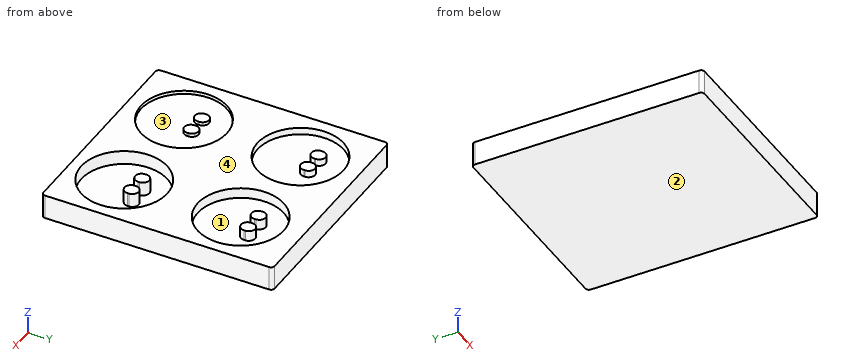
from build123d import *

# Parameters (mm, degrees)
BOSS_EXTRUDE1_DEPTH = 7
CAVITY1_START       = -3
CAVITY1_OUTLINE_R   = 12.36
CAVITY1_DEPTH       = 3
CAVITY1_START_2     = -2
CAVITY1_2_OUTLINE_R = 12.36
CAVITY1_2_DEPTH     = 2
CAVITY1_START_3     = -4
CAVITY1_3_OUTLINE_R = 12.36
CAVITY1_3_DEPTH     = 1
CAVITY1_START_4     = -1
CAVITY1_4_OUTLINE_R = 12.36
CAVITY1_4_DEPTH     = 1


# Read off the part's stored shape, not the designer's step: Cavity1
with BuildPart() as part:
    # Sketch1 → Boss-Extrude1 (new body)
    with BuildSketch(Plane.XY):
        with BuildLine():
            Line((38.123582206, -19.216804324), (-21.063563238, -19.216804324))
            ThreePointArc((-21.063563238, -19.216804324), (-21.770670019, -18.923911105), (-22.063563238, -18.216804324))
            Line((-22.063563238, -18.216804324), (-22.063563238, 46.15189529))
            ThreePointArc((-22.063563238, 46.15189529), (-21.770670019, 46.859002071), (-21.063563238, 47.15189529))
            Line((-21.063563238, 47.15189529), (38.123582206, 47.15189529))
            ThreePointArc((38.123582206, 47.15189529), (38.830688987, 46.859002071), (39.123582206, 46.15189529))
            Line((39.123582206, 46.15189529), (39.123582206, -18.216804324))
            ThreePointArc((39.123582206, -18.216804324), (38.830688987, -18.923911105), (38.123582206, -19.216804324))
        make_face()
    extrude(amount=-BOSS_EXTRUDE1_DEPTH)

    # Cavity1 outline → Cavity1 (cut)
    # profile 1 of 2: a face of its own
    with BuildSketch(Plane.XY.offset(CAVITY1_START)):
        with Locations((23.634896534, -3.890788044)):
            Circle(CAVITY1_OUTLINE_R)
        with BuildLine():
            ThreePointArc((18.999896534, -0.040788044), (20.849896534, 1.809211956), (22.699896534, -0.040788044))
            Line((22.699896534, -0.040788044), (22.699896534, -0.430788044))
            ThreePointArc((22.699896534, -0.430788044), (20.849896534, -2.280788044), (18.999896534, -0.430788044))
            Line((18.999896534, -0.430788044), (18.999896534, -0.040788044))
        make_face(mode=Mode.SUBTRACT)
        with BuildLine():
            ThreePointArc((24.569896534, -0.040788044), (26.419896534, 1.809211956), (28.269896534, -0.040788044))
            Line((28.269896534, -0.040788044), (28.269896534, -0.430788044))
            ThreePointArc((28.269896534, -0.430788044), (26.419896534, -2.280788044), (24.569896534, -0.430788044))
            Line((24.569896534, -0.430788044), (24.569896534, -0.040788044))
        make_face(mode=Mode.SUBTRACT)
    # profile 2 of 2: a face of its own
    with BuildSketch(Plane.XY.offset(CAVITY1_START)):
        with Locations((23.634896534, 29.54740971)):
            Circle(CAVITY1_OUTLINE_R)
        with BuildLine():
            Line((22.699896534, 33.39740971), (22.699896534, 33.00740971))
            ThreePointArc((22.699896534, 33.00740971), (20.849896534, 31.15740971), (18.999896534, 33.00740971))
            Line((18.999896534, 33.00740971), (18.999896534, 33.39740971))
            ThreePointArc((18.999896534, 33.39740971), (20.849896534, 35.24740971), (22.699896534, 33.39740971))
        make_face(mode=Mode.SUBTRACT)
        with BuildLine():
            Line((28.269896534, 33.39740971), (28.269896534, 33.00740971))
            ThreePointArc((28.269896534, 33.00740971), (26.419896534, 31.15740971), (24.569896534, 33.00740971))
            Line((24.569896534, 33.00740971), (24.569896534, 33.39740971))
            ThreePointArc((24.569896534, 33.39740971), (26.419896534, 35.24740971), (28.269896534, 33.39740971))
        make_face(mode=Mode.SUBTRACT)
    extrude(amount=CAVITY1_DEPTH, mode=Mode.SUBTRACT)

    # Cavity1 2 outline → Cavity1 2 (cut)
    with BuildSketch(Plane.XY.offset(CAVITY1_START_2)):
        with Locations((-6.365103466, 30.435007788)):
            Circle(CAVITY1_2_OUTLINE_R)
        with BuildLine():
            ThreePointArc((-11.000103466, 34.285007788), (-9.150103466, 36.135007788), (-7.300103466, 34.285007788))
            Line((-7.300103466, 34.285007788), (-7.300103466, 33.895007788))
            ThreePointArc((-7.300103466, 33.895007788), (-9.150103466, 32.045007788), (-11.000103466, 33.895007788))
            Line((-11.000103466, 33.895007788), (-11.000103466, 34.285007788))
        make_face(mode=Mode.SUBTRACT)
        with BuildLine():
            ThreePointArc((-5.430103466, 34.285007788), (-3.580103466, 36.135007788), (-1.730103466, 34.285007788))
            Line((-1.730103466, 34.285007788), (-1.730103466, 33.895007788))
            ThreePointArc((-1.730103466, 33.895007788), (-3.580103466, 32.045007788), (-5.430103466, 33.895007788))
            Line((-5.430103466, 33.895007788), (-5.430103466, 34.285007788))
        make_face(mode=Mode.SUBTRACT)
    extrude(amount=CAVITY1_2_DEPTH, mode=Mode.SUBTRACT)

    # Cavity1 3 outline → Cavity1 3 (cut)
    with BuildSketch(Plane.XY.offset(CAVITY1_START_3)):
        with Locations((23.634896534, -3.890788044)):
            Circle(CAVITY1_3_OUTLINE_R)
        with BuildLine():
            ThreePointArc((18.999896534, -0.040788044), (20.849896534, 1.809211956), (22.699896534, -0.040788044))
            Line((22.699896534, -0.040788044), (22.699896534, -0.430788044))
            ThreePointArc((22.699896534, -0.430788044), (20.849896534, -2.280788044), (18.999896534, -0.430788044))
            Line((18.999896534, -0.430788044), (18.999896534, -0.040788044))
        make_face(mode=Mode.SUBTRACT)
        with BuildLine():
            ThreePointArc((24.569896534, -0.040788044), (26.419896534, 1.809211956), (28.269896534, -0.040788044))
            Line((28.269896534, -0.040788044), (28.269896534, -0.430788044))
            ThreePointArc((28.269896534, -0.430788044), (26.419896534, -2.280788044), (24.569896534, -0.430788044))
            Line((24.569896534, -0.430788044), (24.569896534, -0.040788044))
        make_face(mode=Mode.SUBTRACT)
    extrude(amount=CAVITY1_3_DEPTH, mode=Mode.SUBTRACT)

    # Cavity1 4 outline → Cavity1 4 (cut)
    with BuildSketch(Plane.XY.offset(CAVITY1_START_4)):
        with Locations((-6.365103466, -3.03425393)):
            Circle(CAVITY1_4_OUTLINE_R)
        with BuildLine():
            Line((-7.300103466, 0.81574607), (-7.300103466, 0.42574607))
            ThreePointArc((-7.300103466, 0.42574607), (-9.150103466, -1.42425393), (-11.000103466, 0.42574607))
            Line((-11.000103466, 0.42574607), (-11.000103466, 0.81574607))
            ThreePointArc((-11.000103466, 0.81574607), (-9.150103466, 2.66574607), (-7.300103466, 0.81574607))
        make_face(mode=Mode.SUBTRACT)
        with BuildLine():
            Line((-1.730103466, 0.81574607), (-1.730103466, 0.42574607))
            ThreePointArc((-1.730103466, 0.42574607), (-3.580103466, -1.42425393), (-5.430103466, 0.42574607))
            Line((-5.430103466, 0.42574607), (-5.430103466, 0.81574607))
            ThreePointArc((-5.430103466, 0.81574607), (-3.580103466, 2.66574607), (-1.730103466, 0.81574607))
        make_face(mode=Mode.SUBTRACT)
    extrude(amount=CAVITY1_4_DEPTH, mode=Mode.SUBTRACT)


solid = part.part
Check sheet for the modelled part. Datum: model origin and axes. Units: mm. Face numbers are marked on the shaded views. A direction names the side the tool comes from. Round coordinates to 2 decimals unless told otherwise and drop trailing zeros. Write each loop counter-clockwise with the first axis right and the second up, starting at its lowest first coordinate (ties: lowest second). Pieces come first, ordered by that corner, then holes. Notation, with made-up numbers: (-0.75, -13) - (42.25, -13) arc R22 ccw to (42.25, 8) - close; hole circle Ø9 at (25, 40). An arc over 180 degrees is marked (long way). Return JSON: item names as keys, results as strings.
Q1. Access from +Z, -Z, +X, -X, +Y, -Y to the whole of each face (thin tool, end or side, straight path). Record for the marked faces 3 and 4.
Returned:
{"face 3": "+Z", "face 4": "+Z, +X, -X, +Y, -Y"}
Q2. Cross-section at D-D (x = -9). Record the boundary of the cut face in (y, z), then the cut area to 3 significant figures.
Returned:
{"outline": "(-19.22, -7) - (47.15, -7) - (47.15, 0) - (42.51, 0) - (42.51, -2) - (36.13, -2) - (36.13, 0) - (32.05, 0) - (32.05, -2) - (18.36, -2) - (18.36, 0) - (9.04, 0) - (9.04, -1) - (2.66, -1) - (2.66, 0) - (-1.42, 0) - (-1.42, -1) - (-15.11, -1) - (-15.11, 0) - (-19.22, 0) - close", "area": "404 mm²"}
Q3. Cross-section at A-A (y = 37.5). Record the boundary of the cut face in (x, z), then the cut area to 3 significant figures.
Returned:
{"outline": "(-22.06, -7) - (39.12, -7) - (39.12, 0) - (33.1, 0) - (33.1, -3) - (14.17, -3) - (14.17, 0) - (3.78, 0) - (3.78, -2) - (-16.51, -2) - (-16.51, 0) - (-22.06, 0) - close", "area": "331 mm²"}
Q4. Depth check by flat-ended pin: P1, Ø12.5, axis at x = -2.5, y = -2, coming from the +Z side; P2, Ø7.5, axis at x = 23, y = -9.5, coming from the +Z side. Enter the tip coordinate at first touch or a pass-through.
Returned:
{"P1": "stops at z = 0", "P2": "stops at z = -4"}
Q5. Scan lines: L1, parallel to X at y = 26, z = -0.25; L2, parallel to Y at x = 15, z = -1.75; L3, parallel to X at y = 6, z = -0.75. Record each from-to range of solid material in increasing order. Write a range as from..to.
Returned:
{"L1": "x = -22.06..-17.9, 5.17..11.79, 35.47..39.12", "L2": "y = -19.22..-12.73, 4.95..20.7, 38.39..47.15", "L3": "x = -22.06..-14.8, 2.07..16.22, 31.05..39.12"}
Q6. Draft check along Y on the marked faces 1 and 2. Enter one of: released by +Y, released by -Y, zero draft, split by the parting line, or undercut.
Returned:
{"face 1": "undercut", "face 2": "zero draft"}
Q7. Cross-section at C-C (x = 0.5). Record the boundary of the cut face in (y, z).
Returned:
{"outline": "(-19.22, -7) - (47.15, -7) - (47.15, 0) - (40.71, 0) - (40.71, -2) - (20.16, -2) - (20.16, 0) - (7.24, 0) - (7.24, -1) - (-13.31, -1) - (-13.31, 0) - (-19.22, 0) - close"}
Q8. Cross-section at B-B (x = 27.5). Record the boundary of the cut face in (y, z), then the cut area to 3 significant figures.
Returned:
{"outline": "(-19.22, -7) - (47.15, -7) - (47.15, 0) - (41.29, 0) - (41.29, -3) - (34.9, -3) - (34.9, 0) - (31.51, 0) - (31.51, -3) - (17.81, -3) - (17.81, 0) - (7.85, 0) - (7.85, -4) - (1.46, -4) - (1.46, 0) - (-1.93, 0) - (-1.93, -4) - (-15.63, -4) - (-15.63, 0) - (-19.22, 0) - close", "area": "324 mm²"}
